Verification items for the finished model (mm, model axes). Face numbers are marked on the shaded views. A direction names the side the tool comes from. Give positions to 0.01 mm unless a question says otherwise; leave off trailing zeros. Loops run counter-clockwise (first coordinate to the right, second up) from the corner with the lowest first, then second, coordinate; pieces in that order, holes last. Notation, with made-up numbers: M -30.5,41.25 L 19.5,41.25 A14 ccw 19.5,46.25 Z; hole C 41.5,3.25 d2. An arc over 180 degrees is marked long. Use CSV: the item, a comma, the result in double quotes.
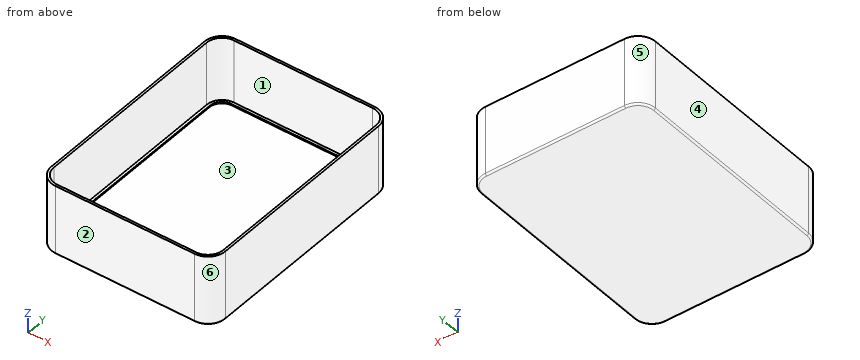
from build123d import *

# Parameters (mm, degrees)
F4_DEPTH = 1.8
F5_DEPTH = 20
F6_DEPTH = 1.4
F7_R     = 0.5


with BuildPart() as f4:
    # F3 (on Top) → F4 (new body)
    with BuildSketch(Plane.XY):
        with BuildLine():
            ThreePointArc((24.35, 28.45), (23.0612698372, 31.5612698372), (19.95, 32.85))
            Line((19.95, 32.85), (-19.95, 32.85))
            ThreePointArc((-19.95, 32.85), (-23.0612698372, 31.5612698372), (-24.35, 28.45))
            Line((-24.35, 28.45), (-24.35, -28.45))
            ThreePointArc((-24.35, -28.45), (-23.0612698372, -31.5612698372), (-19.95, -32.85))
            Line((-19.95, -32.85), (19.95, -32.85))
            ThreePointArc((19.95, -32.85), (23.0612698372, -31.5612698372), (24.35, -28.45))
            Line((24.35, -28.45), (24.35, 28.45))
        make_face()
        with BuildLine():
            Line((20, -32.1), (-20, -32.1))
            ThreePointArc((-20, -32.1), (-22.5455844123, -31.0455844123), (-23.6, -28.5))
            Line((-23.6, -28.5), (-23.6, 28.5))
            ThreePointArc((-23.6, 28.5), (-22.5455844123, 31.0455844123), (-20, 32.1))
            Line((-20, 32.1), (20, 32.1))
            ThreePointArc((20, 32.1), (22.5455844123, 31.0455844123), (23.6, 28.5))
            Line((23.6, 28.5), (23.6, -28.5))
            ThreePointArc((23.6, -28.5), (22.5455844123, -31.0455844123), (20, -32.1))
        make_face(mode=Mode.SUBTRACT)
    extrude(amount=F4_DEPTH)

    # F3 (on Top) → F5 (join)
    with BuildSketch(Plane.XY):
        with BuildLine():
            ThreePointArc((-25, -28.5), (-23.5355339059, -32.0355339059), (-20, -33.5))
            Line((-20, -33.5), (20, -33.5))
            ThreePointArc((20, -33.5), (23.5355339059, -32.0355339059), (25, -28.5))
            Line((25, -28.5), (25, 28.5))
            ThreePointArc((25, 28.5), (23.5355339059, 32.0355339059), (20, 33.5))
            Line((20, 33.5), (-20, 33.5))
            ThreePointArc((-20, 33.5), (-23.5355339059, 32.0355339059), (-25, 28.5))
            Line((-25, 28.5), (-25, -28.5))
        make_face()
        with BuildLine():
            Line((-19.95, 32.85), (19.95, 32.85))
            ThreePointArc((19.95, 32.85), (23.0612698372, 31.5612698372), (24.35, 28.45))
            Line((24.35, 28.45), (24.35, -28.45))
            ThreePointArc((24.35, -28.45), (23.0612698372, -31.5612698372), (19.95, -32.85))
            Line((19.95, -32.85), (-19.95, -32.85))
            ThreePointArc((-19.95, -32.85), (-23.0612698372, -31.5612698372), (-24.35, -28.45))
            Line((-24.35, -28.45), (-24.35, 28.45))
            ThreePointArc((-24.35, 28.45), (-23.0612698372, 31.5612698372), (-19.95, 32.85))
        make_face(mode=Mode.SUBTRACT)
    extrude(amount=F5_DEPTH)

    # F3 (on Top) → F6 (join)
    with BuildSketch(Plane.XY):
        with BuildLine():
            ThreePointArc((-23.6, -28.5), (-22.5455844123, -31.0455844123), (-20, -32.1))
            Line((-20, -32.1), (20, -32.1))
            ThreePointArc((20, -32.1), (22.5455844123, -31.0455844123), (23.6, -28.5))
            Line((23.6, -28.5), (23.6, 28.5))
            ThreePointArc((23.6, 28.5), (22.5455844123, 31.0455844123), (20, 32.1))
            Line((20, 32.1), (-20, 32.1))
            ThreePointArc((-20, 32.1), (-22.5455844123, 31.0455844123), (-23.6, 28.5))
            Line((-23.6, 28.5), (-23.6, -28.5))
        make_face()
    extrude(amount=F6_DEPTH)

    # F7
    f7_edges = [f4.edges().sort_by_distance(p)[0] for p in [
        (25, 0, 0),
    ]]
    fillet(f7_edges, radius=F7_R)


solid = f4.part
(1) Section check A-A on z = 18.75. Record the cut outline in (x, y), plus the area to 3 significant figures.
Calculated:
outline,"M -25,-28.5 A5 ccw -20,-33.5 L 20,-33.5 A5 ccw 25,-28.5 L 25,28.5 A5 ccw 20,33.5 L -20,33.5 A5 ccw -25,28.5 Z; hole M -24.35,-28.45 A4.4 ccw -19.95,-32.85 L 19.95,-32.85 A4.4 ccw 24.35,-28.45 L 24.35,28.45 A4.4 ccw 19.95,32.85 L -19.95,32.85 A4.4 ccw -24.35,28.45 Z"
area,"146 mm²"
(2) Section check B-B on y = 21.5. Record the cut outline in (x, z), plus the area to 3 significant figures.
Calculated:
outline,"M -25,0.5 A0.5 ccw -24.5,0 L 24.5,0 A0.5 ccw 25,0.5 L 25,20 L 24.35,20 L 24.35,1.8 L 23.6,1.8 L 23.6,1.4 L -23.6,1.4 L -23.6,1.8 L -24.35,1.8 L -24.35,20 L -25,20 Z"
area,"94.7 mm²"
(3) Section check C-C on x = 11.5. Record the cut outline in (y, z).
Calculated:
outline,"M -33.5,0.5 A0.5 ccw -33,0 L 33,0 A0.5 ccw 33.5,0.5 L 33.5,20 L 32.85,20 L 32.85,1.8 L 32.1,1.8 L 32.1,1.4 L -32.1,1.4 L -32.1,1.8 L -32.85,1.8 L -32.85,20 L -33.5,20 Z"
(4) Scan lines: L1, parallel to Y at x = 2, z = 8.5; L2, parallel to X at y = 27, z = 2.75; L3, parallel to Z at x = 18.5, y = 29.5. Record each from-to range of solid material in increasing order. Write a range as from..to.
Calculated:
L1,"y = -33.5..-32.85, 32.85..33.5"
L2,"x = -25..-24.35, 24.35..25"
L3,"z = 0..1.4"
(5) Mould release check, pull along Y, two halves, no side actions. Record for the marked faces 3, 4, 5 and 6: released by +Y, released by -Y, zero draft, split by the parting line, or undercut.
Calculated:
face 3,"undercut"
face 4,"zero draft"
face 5,"released by +Y"
face 6,"released by -Y"
(6) Tool access check on the marked faces 1 and 2. Record the directions out of +Z, -Z, +X, -X, +Y, -Y that give a thin tool (end or side, any length) a straight path to the whole face; none if there is none.
Calculated:
face 1,"+Z"
face 2,"+Z, -Z, +X, -X, -Y"
(7) Depth check by flat-ended pin: pin 1 Ø4 at (x, y) = (7.5, 8.5) entering from +Z. Enter the tip coordinate at first touch or a pass-through.
Calculated:
pin 1,"stops at z = 1.4"
